Part print with two shaded views. Sizes in mm from the minimum x, y, z corner. A direction names the side the tool comes from. Give positions to 0.01 mm unless a question says otherwise; leave off trailing zeros. Order: outer loops, then holes, each group sorted by start corner. A loop starts at its lowest first (then second) coordinate and runs counter-clockwise, first axis right, second up.
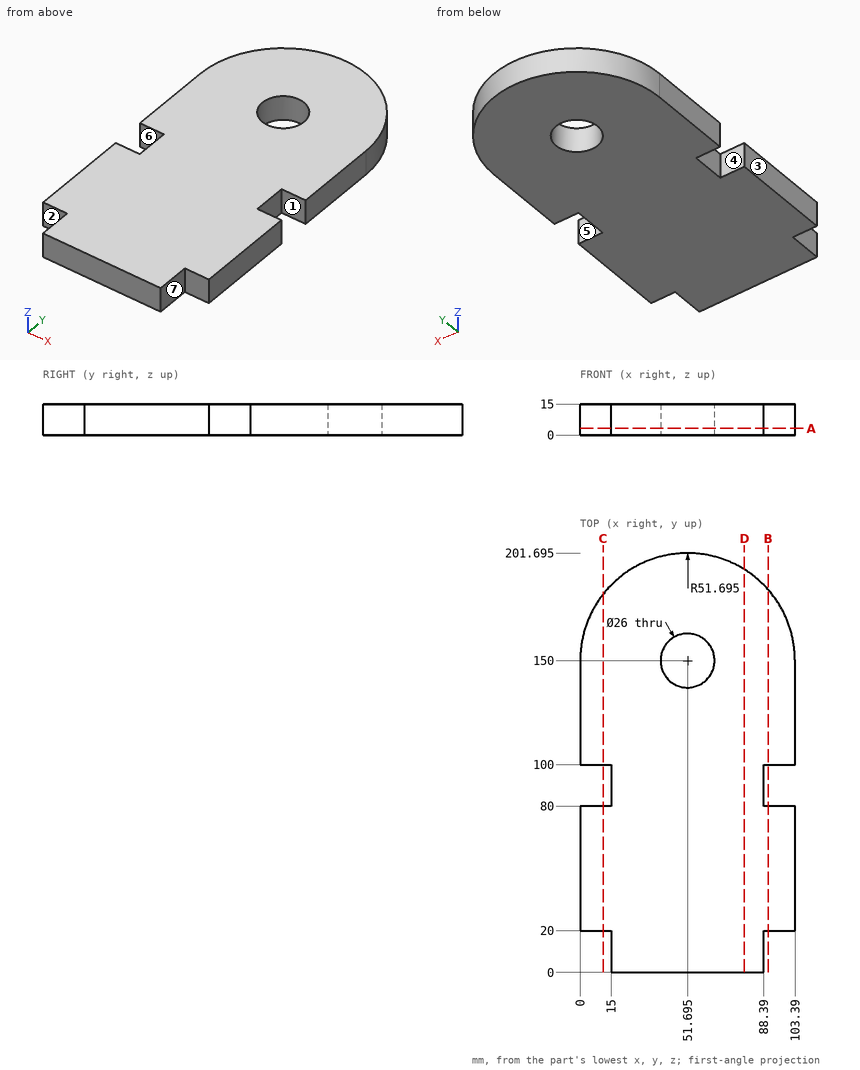
1. Mould opens along Y. For the marked faces 1, 2, 3 and 4 say: released by +Y, released by -Y, zero draft, split by the parting line, or undercut.
2. 3-axis set-ups, long thin cutter, end or side, ignore diameter. For the marked faces 5, 6 and 7: which of +Z, -Z, +X, -X, +Y, -Y reach the whole face in a straight line?
3. Pin check, flat tips, straight feed: P1, Ø7.5, axis at x = 95.5, z = 8.5, coming from the +Y side; P2, Ø23.5, axis at x = 51.695, y = 150, coming from the +Z side; P3, Ø8, axis at y = 99.5, z = 12, coming from the -X side; P4, Ø7.5, axis at x = 9, z = 6, coming from the +Y side (3 decimals). Stop position of each tip, or through.
4. Saw through at B-B on x = 90.5. Give the cut face in (y, z).
5. Saw through at A-A on z = 3.25. Give the cut face in (x, y) (3 decimals).
6. Saw through at C-C on x = 11. Give the cut face in (y, z), plus the area to 3 significant figures.
7. Wall check: line 1 (X direction, y = 15.5, z = 2); line 2 (Y direction, x = 12, z = 6); line 3 (Y direction, x = 57, z = 7). Give the ranges that are in metal, low to high.
8. Saw through at D-D on x = 79. Give the cut face in (y, z).
Reported:
1. face 1: undercut
1. face 2: released by -Y
1. face 3: zero draft
1. face 4: undercut
2. face 5: +Z, -Z, +X
2. face 6: +Z, -Z, -X
2. face 7: +Z, -Z, +X, -Y
3. P1: stops at y = 182.68
3. P2: passes through
3. P3: stops at x = 0
3. P4: stops at y = 183.995
4. outline: (20, 0) - (80, 0) - (80, 15) - (20, 15) - close; (100, 0) - (184.15, 0) - (184.15, 15) - (100, 15) - close
5. outline: (0, 20) - (15, 20) - (15, 0) - (88.39, 0) - (88.39, 20) - (103.39, 20) - (103.39, 80) - (88.39, 80) - (88.39, 100) - (103.39, 100) - (103.39, 150) arc R51.695 ccw to (0, 150) - (0, 100) - (15, 100) - (15, 80) - (0, 80) - close; hole circle Ø26 at (51.695, 150)
6. outline: (20, 0) - (80, 0) - (80, 15) - (20, 15) - close; (100, 0) - (181.88, 0) - (181.88, 15) - (100, 15) - close
6. area: 2,130 mm2
7. line 1: x = 15 to 88.39
7. line 2: y = 20 to 80, 100 to 183.12
7. line 3: y = 0 to 138.13, 161.87 to 201.42
8. outline: (0, 0) - (193.9, 0) - (193.9, 15) - (0, 15) - close
